Geometry: final body of the model. Coordinates: model frame, mm. Give positions to 0.01 mm unless a question says otherwise; leave off trailing zeros. One line per item, written item: value.
```python
from build123d import *

# Parameters (mm, degrees)
SKETCH1_W           = 402
SKETCH1_H           = 50
SKETCH1_R           = 6
SKETCH1_R_2         = 1.8
SKETCH1_R_3         = 11
SKETCH1_R_4         = 1.6
SKETCH1_R_5         = 2.6
BOSS_EXTRUDE1_DEPTH = 8


with BuildPart() as part:
    # Sketch1 → Boss-Extrude1 (new body)
    with BuildSketch(Plane.XY):
        Rectangle(SKETCH1_W, SKETCH1_H)
        with Locations((-178, 0)):
            Circle(SKETCH1_R, mode=Mode.SUBTRACT)
        with Locations((168, 0)):
            Circle(SKETCH1_R_2, mode=Mode.SUBTRACT)
        Circle(SKETCH1_R_3, mode=Mode.SUBTRACT)
        with Locations((-188, 0)):
            Circle(SKETCH1_R_2, mode=Mode.SUBTRACT)
        with Locations((-168, 0)):
            Circle(SKETCH1_R_2, mode=Mode.SUBTRACT)
        with Locations((188, 0)):
            Circle(SKETCH1_R_2, mode=Mode.SUBTRACT)
        with Locations((178, 0)):
            Circle(SKETCH1_R, mode=Mode.SUBTRACT)
        with Locations((-15.5, 15.5)):
            Circle(SKETCH1_R_4, mode=Mode.SUBTRACT)
        with Locations((15.5, 15.5)):
            Circle(SKETCH1_R_4, mode=Mode.SUBTRACT)
        with Locations((-15.5, -15.5)):
            Circle(SKETCH1_R_4, mode=Mode.SUBTRACT)
        with Locations((15.5, -15.5)):
            Circle(SKETCH1_R_4, mode=Mode.SUBTRACT)
        with Locations((0, 17)):
            Circle(SKETCH1_R_5, mode=Mode.SUBTRACT)
        with Locations((40, 17)):
            Circle(SKETCH1_R_5, mode=Mode.SUBTRACT)
        with Locations((80, 17)):
            Circle(SKETCH1_R_5, mode=Mode.SUBTRACT)
        with Locations((120, 17)):
            Circle(SKETCH1_R_5, mode=Mode.SUBTRACT)
        with Locations((160, 17)):
            Circle(SKETCH1_R_5, mode=Mode.SUBTRACT)
        with Locations((-40, 17)):
            Circle(SKETCH1_R_5, mode=Mode.SUBTRACT)
        with Locations((-80, 17)):
            Circle(SKETCH1_R_5, mode=Mode.SUBTRACT)
        with Locations((-120, 17)):
            Circle(SKETCH1_R_5, mode=Mode.SUBTRACT)
        with Locations((-160, 17)):
            Circle(SKETCH1_R_5, mode=Mode.SUBTRACT)
    extrude(amount=BOSS_EXTRUDE1_DEPTH)


solid = part.part
```
1) Section A-A, the plane z = 5. Count the separate pieces of the cut face and the enclosed holes in it, then the cut area to 3 significant figures.
Answers below:
separate pieces: 1
enclosed holes: 20
area: 19,200 mm^2
2) Mould query, pull axis Y, two halves, no side actions, for faces 1 (the face through (-184, 0, 4)), 2 (the face through (-3, 25, 4)), 3 (the face through (201, 0, 4)). Classes: released by +Y, released by -Y, zero draft, split by the parting line, or undercut.
Answers below:
face 1: undercut
face 2: released by +Y
face 3: zero draft
3) Material intervals for line 1 along Y through (x, z) = (15.5, 4); line 2 along Y through (x, z) = (0, 6); line 3 along Y through (x, z) = (160, 2.75), sorted ascending.
Answers below:
line 1: -25 to -17.1, -13.9 to 13.9, 17.1 to 25
line 2: -25 to -11, 11 to 14.4, 19.6 to 25
line 3: -25 to 14.4, 19.6 to 25
